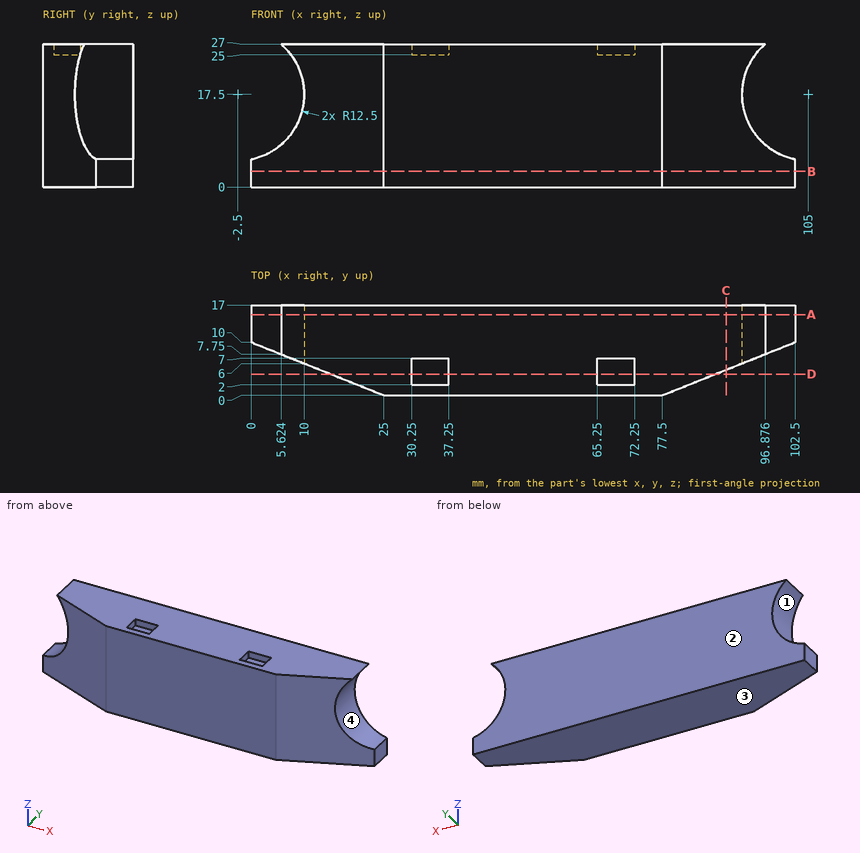
Study the drawing (mm; zero at the part's minimum x, y, z) and answer. Round coordinates to 2 decimals unless told otherwise and drop trailing zeros. Write each loop counter-clockwise with the first axis right and the second up, starting at its lowest first coordinate (ties: lowest second). Pieces come first, ordered by that corner, then holes. Notation, with made-up numbers: (-13, 12) - (2, 12) arc R14 ccw to (2, 19) - close; hole circle Ø3 at (-11.5, 83). An arc over 180 degrees is marked (long way). Use a Markdown table: item, result. Add a question column.
1. The part is cut by section B-B (z = 3). Write down the section's boundary in (x, y), and give its area (3 significant figures).
2. The part is cut by section D-D (y = 4). Write down the section's boundary in (x, z), and give its area (3 significant figures).
3. Flat-ended cylindrical pins translate along their axes: P1, Ø3, axis at y = 5, z = 14.5, coming from the -X side (1 decimal); P2, Ø10, axis at y = 7.5, z = 13, coming from the -X side; P3, Ø4, axis at y = 4.5, z = 13.5, coming from the -X side; P4, Ø1.6, axis at x = 33, z = 26.5, coming from the -Y side. Find the tip coordinate at first contact, or state that the pin passes through.
4. The part is cut by section C-C (x = 89.5). Write down the section's boundary in (y, z).
5. For a pull along Z with two mould halves and no side action, classify the marked faces 1, 2, 3 and 4 as +Z half, -Z half, draft (parallel to the pull), parting line (faces both ways), or undercut.
6. The part is cut by section A-A (y = 15.25). Write down the section's boundary in (x, z), and give its area (3 significant figures).
7. Consider line 1 (X direction, y = 12, z = 17); line 2 (Z direction, x = 7, y = 15) (1 decimal); line 3 (Y direction, x = 82.5, z = 7.25). Determine where each line is inside the solid, lowest interval first.
Reported:
| question | item | result |
|---|---|---|
| 1 | outline | (0, 10) - (25, 0) - (77.5, 0) - (102.5, 10) - (102.5, 17) - (0, 17) - close |
| 1 | area | 1,490 mm^2 |
| 2 | outline | (15, 0) - (87.5, 0) - (87.5, 27) - (72.25, 27) - (72.25, 25) - (65.25, 25) - (65.25, 27) - (37.25, 27) - (37.25, 25) - (30.25, 25) - (30.25, 27) - (15, 27) - close |
| 2 | area | 1,930 mm^2 |
| 3 | P1 | x = 9.4 |
| 3 | P2 | x = 5.63 |
| 3 | P3 | x = 9.08 |
| 3 | P4 | y = 0 |
| 4 | outline | (4.8, 0) - (17, 0) - (17, 27) - (4.8, 27) - close |
| 5 | face 1 | undercut |
| 5 | face 2 | draft |
| 5 | face 3 | -Z half |
| 5 | face 4 | undercut |
| 6 | outline | (0, 0) - (102.5, 0) - (102.5, 5.25) arc R12.5 cw to (96.88, 27) - (5.62, 27) arc R12.5 cw to (0, 5.25) - close |
| 6 | area | 2,420 mm^2 |
| 7 | line 1 | 9.99 to 92.51 |
| 7 | line 2 | 0 to 9.4, 25.6 to 27 |
| 7 | line 3 | 2 to 17 |
